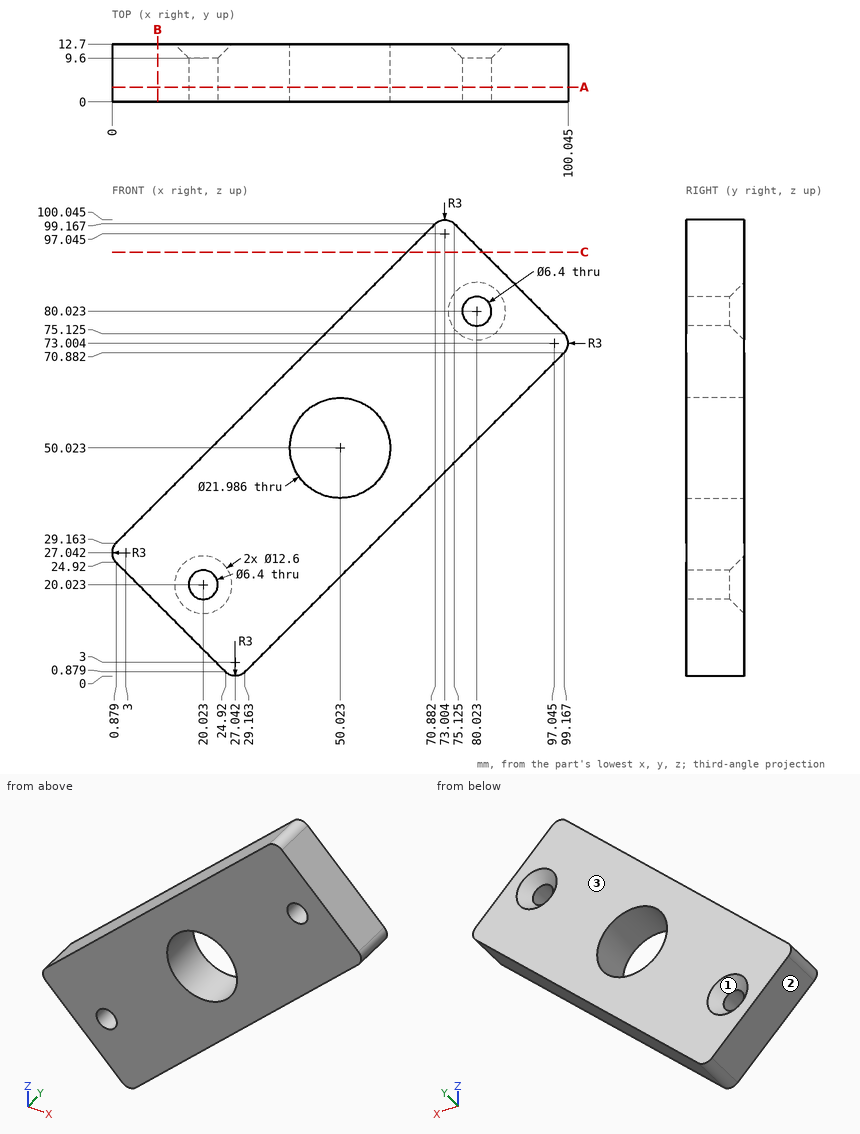
The figure shows three views and two pictorial views of one solid part (mm, origin at its lowest corner). Answer the questions. Coordinates: 2 decimals unless noted, no trailing zeros. Loops run counter-clockwise (first coordinate to the right, second up) from the corner with the lowest first, then second, coordinate; pieces in that order, holes last. Notation, with made-up numbers: (77, 76.5) - (100, 76.5) arc R18 ccw to (100, 105.5) - close; hole circle Ø4 at (-16.5, 25.5). An arc over 180 degrees is marked (long way). Write item = value, one per line.
1) Each of these flat-tipped pins is pushed along its axis until it touches: P1, Ø1.5, axis at x = 51.5, y = 9, coming from the -Z side (1 decimal); P2, Ø8.5, axis at x = 80.02, z = 80.02, coming from the -Y side; P3, Ø5, axis at y = 6.5, z = 32, coming from the -X side (1 decimal); P4, Ø7.5, axis at x = 20.02, z = 20.02, coming from the +Y side (1 decimal). Where does it stop, or does it pass through?
Responses:
P1 = 22.5
P2 = 0
P3 = 1.2
P4 = 10.2
2) Section B-B (x = 10) is taken. Determine the outline of the cut face in (y, z) (1 decimal).
Responses:
outline = (0, 15.8) - (12.7, 15.8) - (12.7, 38.3) - (0, 38.3) - close
3) Section C-C (z = 93) is taken. Determine the outline of the cut face in (x, y) (1 decimal).
Responses:
outline = (64.7, 0) - (81.3, 0) - (81.3, 12.7) - (64.7, 12.7) - close
4) Section A-A (y = 3.25) is taken. Determine the outline of the cut face in (x, z) (1 decimal), plus the area to 3 significant figures.
Responses:
outline = (0.9, 24.9) - (24.9, 0.9) arc R3 ccw to (29.2, 0.9) - (99.2, 70.9) arc R3 ccw to (99.2, 75.1) - (75.1, 99.2) arc R3 ccw to (70.9, 99.2) - (0.9, 29.2) arc R3 ccw to start; hole circle Ø6.4 at (20, 20); hole circle Ø22 at (50, 50); hole circle Ø6.4 at (80, 80)
area = 3,750 mm^2
5) Determine the mould class of the marked faces 1, 2 and 3 for opening direction X: pulls with the +X half, pulls with the -X half, needs draft (parallel to the pull), parting line crosses it, or undercut.
Responses:
face_1 = undercut
face_2 = pulls with the -X half
face_3 = needs draft
6) Find the intervals of material crossed by line 1 along Z through (x, y) = (17.5, 9.25) (1 decimal); line 2 along Z through (x, y) = (18.5, 5.75) (1 decimal); line 3 along Z through (x, y) = (30, 8) (1 decimal), in increasing order.
Responses:
line_1 = 8.3 to 18.1, 22 to 45.8
line_2 = 7.3 to 17.2, 22.8 to 46.8
line_3 = 1.7 to 58.3
